The model under review builds one solid part; all positions refer to its coordinate system, in mm. A direction names the side the tool comes from. Round coordinates to 2 decimals unless told otherwise and drop trailing zeros. Order: outer loops, then holes, each group sorted by start corner. A loop starts at its lowest first (then second) coordinate and runs counter-clockwise, first axis right, second up. Notation, with made-up numbers: M 33.5,87 L 61.5,87 A33 cw 61.5,118 Z; hole C -2,62 d8. An arc over 180 degrees is marked long. Use a Markdown table: item, result. Add a question column.
1. Consider section B-B on y = -1.5. State the section outline as (x, z) points, then the cut area to 3 significant figures.
2. Consider section A-A on z = -5. State the section outline as (x, y) points (3 decimals), then the cut area to 3 significant figures.
3. The part is to be moulded in two halves that separate along Z. For faces 6 (the flat face through (-26, 18.415, -3)), 7 (the flat face through (23.49, 3.39, 0.64)), 8 (the flat face through (-23.5, 12, -3.175)), 9 (the flat face through (-23.5, 3.39, 0.63)), say which applies: +Z half, -Z half, draft (parallel to the pull), parting line (faces both ways), or undercut.
4. Consider section C-C on x = -14. State the section outline as (y, z) points (3 decimals), then the cut area to 3 significant figures.
5. Consider section D-D on x = 19. State the section outline as (y, z) points (3 decimals), then the cut area to 3 significant figures.
6. To check wall thickness, follow probe 1 along X at (y, z) = (-12, -8.25); probe 2 along X at (y, z) = (17, -2); probe 3 along Y at (x, z) = (-21.5, -5.25) (3 decimals). State the ranges of each line that lie inside material, in increasing order.
7. For faces 1 (the flat face through (0, -13, -12.7)), 2 (the flat face through (0, -18.415, -3)), 3 (the flat face through (-22.86, 3, 4)), 4 (the cylindrical face through (18.321, -7.625, -8.004)), 5 (the flat face through (23.2, -12.4, -3.175)), list the 3-axis set-ups (+Z, -Z, +X, -X, +Y, -Y) from which the entire face can be reached by the end or side of a thin tool; tool diameter is ignored.
8. Insertion check: P1, Ø1.8, axis at x = -22.86, y = 12.065, coming from the -Z side (3 decimals); P2, Ø9.5, axis at x = 5.5, z = 1, coming from the +Y side (3 decimals); P3, Ø3, axis at x = 19.5, y = -10, coming from the +Z side (3 decimals). Each pin has a flat end and moves straight along its axis. Give the tip position at first contact, or say it passes through.
from build123d import *

# Parameters (mm, degrees)
F1_DEPTH      = 6.35
F1_DEPTH_BACK = 12.7
F3_DEPTH      = 30.48
F5_DEPTH      = 9.525
F6_R          = 1.5
F7_DEPTH      = 9.525


with BuildPart() as f1:
    # F0 (on Top) → F1 (new body, two sides)
    with BuildSketch(Plane.XY) as f1_sk:
        Polygon((-29.2099994576, 18.4149997288), (-29.2099994576, -18.4149997288), (29.2099994576, -18.4149997288), (29.2099994576, 18.4149997288), (22.86, 18.4149997288), (22.86, -12.0650002712), (-22.86, -12.0650002712), (-22.86, 18.4149997288), align=None)
    extrude(amount=F1_DEPTH)
    extrude(f1_sk.sketch, amount=-F1_DEPTH_BACK)

    # F2 (on face) → F3 (cut)
    with BuildSketch(Plane(origin=(0, 18.4149997288, 0), x_dir=(-1, 0, 0), z_dir=(0, 1, 0))):
        Polygon((0, 24.13), (-24.13, 0), (0, -24.13), (22.86, -1.27), (22.86, 1.27), align=None)
        Polygon((24.13, 0), (22.86, 1.27), (22.86, -1.27), align=None)
    extrude(amount=-F3_DEPTH, mode=Mode.SUBTRACT)

    # F4 (on face) → F5 (join)
    with BuildSketch(Plane(origin=(0, 0, -12.7), x_dir=(1, 0, 0), z_dir=(0, 0, -1))):
        with BuildLine():
            Line((-22.86, -5.7149997288), (-22.86, -18.4149997288))
            ThreePointArc((-22.86, -18.4149997288), (-18.3698719395, -16.5551277893), (-16.51, -12.0649997288))
            ThreePointArc((-16.51, -12.0649997288), (-18.3698719395, -7.5748716683), (-22.86, -5.7149997288))
        make_face()
        with BuildLine():
            Line((22.86, 12.0650002712), (16.51, 12.0650002712))
            ThreePointArc((16.51, 12.0650002712), (18.3698719395, 7.5748722107), (22.86, 5.7150002712))
            Line((22.86, 5.7150002712), (22.86, 12.0650002712))
        make_face()
    extrude(amount=-F5_DEPTH)

    # F6 (on face) → F7 (cut)
    with BuildSketch(Plane(origin=(0, 0, -12.7), x_dir=(1, 0, 0), z_dir=(0, 0, -1))):
        with Locations((22.86, 12.0650002712)):
            Circle(F6_R)
        with Locations((-22.86, -12.0649997288)):
            Circle(F6_R)
    extrude(amount=-F7_DEPTH, mode=Mode.SUBTRACT)


solid = f1.part
Answer block:
| question | item | result |
|---|---|---|
| 1 | outline | M -29.21,-12.7 L -22.86,-12.7 L -22.86,-1.27 L -24.13,0 L -22.86,1.27 L -22.86,6.35 L -29.21,6.35 Z; M 22.86,-12.7 L 29.21,-12.7 L 29.21,6.35 L 22.86,6.35 L 22.86,1.27 L 24.13,0 L 22.86,-1.27 Z |
| 1 | area | 239 mm^2 |
| 2 | outline | M -29.21,-18.415 L 29.21,-18.415 L 29.21,18.415 L 22.86,18.415 L 22.86,-5.715 A6.35 ccw 16.51,-12.065 L -22.86,-12.065 L -22.86,5.715 A6.35 ccw -22.86,18.415 L -29.21,18.415 Z; hole C -22.86,12.065 d3; hole C 22.86,-12.065 d3 |
| 2 | area | 839 mm^2 |
| 3 | face 6 | draft |
| 3 | face 7 | undercut |
| 3 | face 8 | -Z half |
| 3 | face 9 | undercut |
| 4 | outline | M -18.415,-12.7 L -12.065,-12.7 L -12.065,6.35 L -18.415,6.35 Z |
| 4 | area | 121 mm^2 |
| 5 | outline | M -18.415,-12.7 L -7.023,-12.7 L -7.023,-3.175 L -12.065,-3.175 L -12.065,6.35 L -18.415,6.35 Z |
| 5 | area | 169 mm^2 |
| 6 | probe 1 | -29.21 to -22.86, 16.51 to 21.36, 24.36 to 29.21 |
| 6 | probe 2 | -29.21 to -22.86, 22.86 to 29.21 |
| 6 | probe 3 | -18.415 to -12.065, 5.862 to 11.432, 12.698 to 18.268 |
| 7 | face 1 | -Z, +X, -X, +Y, -Y |
| 7 | face 2 | +Z, -Z, +X, -X, -Y |
| 7 | face 3 | +Z, +Y |
| 7 | face 4 | +Z, -Z, +Y |
| 7 | face 5 | -Z |
| 8 | P1 | z = -3.175 |
| 8 | P2 | y = -12.065 |
| 8 | P3 | z = -3.175 |
